The listing builds one solid part. Answer for the finished solid, in the listing's coordinates (mm). A direction names the side the tool comes from. Round coordinates to 2 decimals unless told otherwise and drop trailing zeros. Loops run counter-clockwise (first coordinate to the right, second up) from the corner with the lowest first, then second, coordinate; pieces in that order, holes last. Notation, with made-up numbers: (-24, 54) -> (15, 54) arc R27 ccw to (15, 71) -> close; hole circle Ø9 at (89.25, -17.5). An arc over 180 degrees is marked (long way). Use a Markdown table: item, result. Add a question column.
Q1. Section A-A on x = 69.5 is taken. Give the vertices of the cut face in (y, z), then the cut area to 3 significant figures.
Q2. Section C-C on y = 1.75 is taken. Give the vertices of the cut face in (x, z).
Q3. For a pull along X with two mould halves and no side action, classify faces 1 (the flat face through (74, -5, -51)), 2 (the flat face through (147, 4, -96)), 3 (the flat face through (150.5, 0, -49)), 4 (the flat face through (0, 0, -49)) as released by +X, released by -X, zero draft, split by the parting line, or undercut.
Q4. Which of the six approach directions +Z, -Z, +X, -X, +Y, -Y give full straight-line access (tool end or side, diameter ignored) to faces 5 (the flat face through (74, 0, -51)), 6 (the flat face through (74, 0, 0))?
Q5. Section B-B on z = -47 is taken. Give the vertices of the cut face in (x, y).
Q6. Given pin 1 Ø8 at (x, z) = (88, -61.5) entering from +Y; pin 2 Ø0.5 at (x, z) = (147.5, -96.5) entering from +Y; pin 3 Ø1 at (x, z) = (2.5, -97.5) entering from +Y, each flat-ended and moving along its own axis, determine where each tip first touches the part or whether it passes through.
Q7. Consider line 1 (X direction, y = 1, z = -85.5); line 2 (Z direction, x = 98, y = 1.5); line 3 (Y direction, x = 9, z = -50). Determine where each line is inside the solid, lowest interval first.
from build123d import *

# Parameters (mm, degrees)
SKETCH1_W           = 150.5
SKETCH1_H           = 100
BOSS_EXTRUDE1_DEPTH = 5
SKETCH2_W           = 138.5
SKETCH2_H           = 91
CUT_EXTRUDE1_DEPTH  = 5
SKETCH3_R           = 1.75
CUT_EXTRUDE2_DEPTH  = 1
SKETCH4_R           = 0.5
CUT_EXTRUDE3_DEPTH  = 5


with BuildPart() as part:
    # Sketch1 → Boss-Extrude1 (new, symmetric)
    with BuildSketch(Plane(origin=(0, 0, 0), x_dir=(1, 0, 0), z_dir=(0, 1, 0))):
        with Locations((75.25, 50)):
            Rectangle(SKETCH1_W, SKETCH1_H)
    extrude(amount=BOSS_EXTRUDE1_DEPTH, both=True)

    # Sketch2 → Cut-Extrude1 (cut)
    with BuildSketch(Plane(origin=(0, 5, 0), x_dir=(1, 0, 0), z_dir=(0, 1, 0))):
        with Locations((75.25, 50)):
            Rectangle(SKETCH2_W, SKETCH2_H)
    extrude(amount=-CUT_EXTRUDE1_DEPTH, mode=Mode.SUBTRACT)

    # Sketch3 → Cut-Extrude2 (cut)
    with BuildSketch(Plane(origin=(0, 5, 0), x_dir=(1, 0, 0), z_dir=(0, 1, 0))):
        with Locations(Location((3.159079735, 96.662135708, 0), (0, 0, 270))):
            Circle(SKETCH3_R)
        with Locations(Location((3.102788334, 3.254527641, 0), (0, 0, 270))):
            Circle(SKETCH3_R)
        with Locations(Location((147.430623058, 3.436900869, 0), (0, 0, 270))):
            Circle(SKETCH3_R)
        with Locations(Location((147.430623058, 96.662135708, 0), (0, 0, 270))):
            Circle(SKETCH3_R)
    extrude(amount=-CUT_EXTRUDE2_DEPTH, mode=Mode.SUBTRACT)

    # Sketch4 → Cut-Extrude3 (cut)
    with BuildSketch(Plane(origin=(0, 4, 0), x_dir=(1, 0, 0), z_dir=(0, 1, 0))):
        with Locations(Location((3.212524906, 96.64723106, 0), (0, 0, 270))):
            Circle(SKETCH4_R)
        with Locations(Location((3.17577296, 3.128534438, 0), (0, 0, 270))):
            Circle(SKETCH4_R)
        with Locations(Location((147.423404744, 3.438562915, 0), (0, 0, 270))):
            Circle(SKETCH4_R)
        with Locations(Location((147.430623058, 96.662135708, 0), (0, 0, 270))):
            Circle(SKETCH4_R)
    extrude(amount=-CUT_EXTRUDE3_DEPTH, mode=Mode.SUBTRACT)


solid = part.part
Checked values:
| question | item | result |
|---|---|---|
| 1 | outline | (-5, -100) -> (5, -100) -> (5, -95.5) -> (0, -95.5) -> (0, -4.5) -> (5, -4.5) -> (5, 0) -> (-5, 0) -> close |
| 1 | area | 545 mm2 |
| 2 | outline | (0, -100) -> (150.5, -100) -> (150.5, 0) -> (0, 0) -> close; hole circle Ø1 at (3.18, -3.13); hole circle Ø1 at (3.21, -96.65); hole (6, -95.5) -> (144.5, -95.5) -> (144.5, -4.5) -> (6, -4.5) -> close; hole circle Ø1 at (147.42, -3.44); hole circle Ø1 at (147.43, -96.66) |
| 3 | face 1 | zero draft |
| 3 | face 2 | undercut |
| 3 | face 3 | released by +X |
| 3 | face 4 | released by -X |
| 4 | face 5 | +Y |
| 4 | face 6 | +Z, +X, -X, +Y, -Y |
| 5 | outline | (0, -5) -> (150.5, -5) -> (150.5, 5) -> (144.5, 5) -> (144.5, 0) -> (6, 0) -> (6, 5) -> (0, 5) -> close |
| 6 | pin 1 | stops at y = 0 |
| 6 | pin 2 | stops at y = -1 |
| 6 | pin 3 | stops at y = 4 |
| 7 | line 1 | x = 0 to 6, 144.5 to 150.5 |
| 7 | line 2 | z = -100 to -95.5, -4.5 to 0 |
| 7 | line 3 | y = -5 to 0 |
